Print and shaded views of the part. All mm, measured from the part's lowest x, y and z. Coordinates: 2 decimals unless noted, no trailing zeros. Order: outer loops, then holes, each group sorted by start corner. A loop starts at its lowest first (then second) coordinate and runs counter-clockwise, first axis right, second up. Notation, with made-up numbers: M -20,50.25 L 13,50.25 A23 ccw 13,64.25 Z; hole C 88.5,-25 d8. An arc over 180 degrees is marked long. One line per item, written item: value.
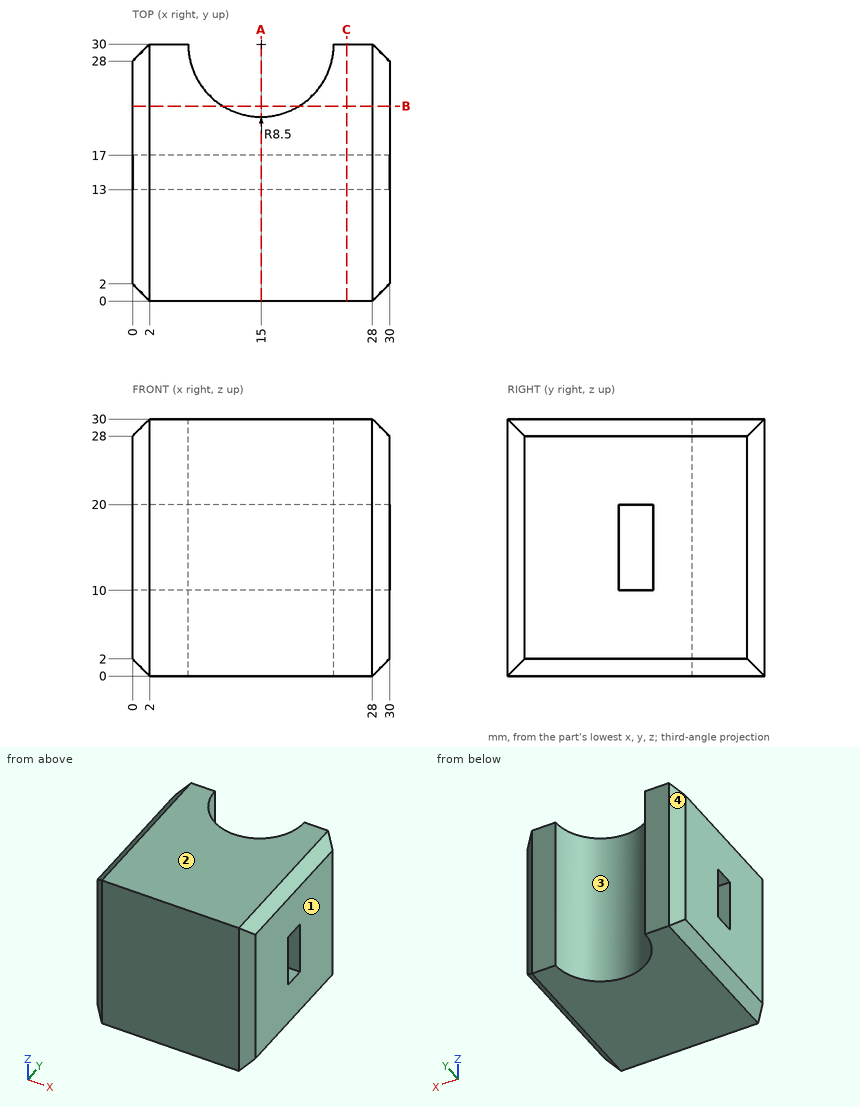
Q1. Slice it at B-B (y = 22.75). List the corners of the cut face in (x, z).
Recorded:
outline: M 0,2 L 2,0 L 10.56,0 L 10.56,30 L 2,30 L 0,28 Z; M 19.44,0 L 28,0 L 30,2 L 30,28 L 28,30 L 19.44,30 Z
Q2. Pin check, flat tips, straight feed: pin 1 Ø8 at (x, z) = (11.5, 12.5) entering from +Y; pin 2 Ø1.5 at (x, z) = (19.5, 17) entering from +Y. Stop position of each tip, or through.
Recorded:
pin 1: stops at y = 26
pin 2: stops at y = 23.32
Q3. Drill centre lines: line 1 along Z through (x, y) = (20.75, 15.75); line 2 along Y through (x, z) = (22.5, 11.25); line 3 along X through (y, z) = (27.5, 20.75). Where is each one in solid material? Low to high.
Recorded:
line 1: z = 0 to 10, 20 to 30
line 2: y = 0 to 13, 17 to 26
line 3: x = 0 to 6.88, 23.12 to 30
Q4. Mould opens along X. For the marked faces 1, 2, 3 and 4 say: released by +X, released by -X, zero draft, split by the parting line, or undercut.
Recorded:
face 1: released by +X
face 2: zero draft
face 3: undercut
face 4: released by -X
Q5. Slice it at C-C (x = 25). List the corners of the cut face in (y, z).
Recorded:
outline: M 0,0 L 30,0 L 30,30 L 0,30 Z; hole M 13,10 L 17,10 L 17,20 L 13,20 Z
Q6. Slice it at A-A (x = 15). List the corners of the cut face in (y, z).
Recorded:
outline: M 0,0 L 21.5,0 L 21.5,30 L 0,30 Z; hole M 13,10 L 17,10 L 17,20 L 13,20 Z
